Could you check a few things on this model? Use its own coordinates, in mm. Face numbers are marked on the shaded views. A direction names the side the tool comes from. Round coordinates to 2 decimals unless told otherwise and drop trailing zeros. Write each loop counter-clockwise with the first axis right and the second up, starting at its lowest first coordinate (ties: lowest second). Pieces come first, ordered by that corner, then holes. Notation, with made-up numbers: (-30, 53) -> (-1, 53) arc R30 ccw to (-1, 83) -> close; hole circle Ø8 at (82.25, -32.75). An arc over 180 degrees is marked (long way). Answer in a Markdown table with one row per item.
from build123d import *

# Parameters (mm, degrees)
BOSS_EXTRU_1_DEPTH      = 2
ESQUISSE3_R             = 1.5
ENL_V_MAT_EXTRU_1_DEPTH = 2
BOSS_EXTRU_2_START      = -2
ESQUISSE4_R             = 1.4
BOSS_EXTRU_2_DEPTH      = 2
ESQUISSE5_R             = 1.6
BOSS_EXTRU_3_DEPTH      = 1
ESQUISSE6_W             = 4
ESQUISSE6_H             = 1
ENL_V_MAT_EXTRU_2_DEPTH = 3


with BuildPart() as part:
    # Esquisse2 → Boss.-Extru.1 (new body)
    with BuildSketch(Plane.XY):
        with BuildLine():
            Line((-2.010396268, -6.486037297), (-15.087524479, 11.205449858))
            ThreePointArc((-15.087524479, 11.205449858), (-14.563165508, 14.701883422), (-11.066731944, 14.177524451))
            Line((-11.066731944, 14.177524451), (2.010396268, -3.513962703))
            ThreePointArc((2.010396268, -3.513962703), (1.486037297, -7.010396268), (-2.010396268, -6.486037297))
        make_face()
    extrude(amount=BOSS_EXTRU_1_DEPTH)

    # Esquisse3 → Enlèv. mat.-Extru.1 (cut)
    with BuildSketch(Plane.XY.offset(2)):
        with Locations((0, -5)):
            Circle(ESQUISSE3_R)
    extrude(amount=-ENL_V_MAT_EXTRU_1_DEPTH, mode=Mode.SUBTRACT)

    # Esquisse4 → Boss.-Extru.2 (add)
    with BuildSketch(Plane.XY.offset(2).offset(BOSS_EXTRU_2_START)):
        with Locations((-13.077128211, 12.691487155)):
            Circle(ESQUISSE4_R)
    extrude(amount=-BOSS_EXTRU_2_DEPTH)

    # Esquisse5 → Boss.-Extru.3 (add)
    with BuildSketch(Plane(origin=(0, 0, -2), x_dir=(-1, 0, 0), z_dir=(0, 0, -1))):
        with Locations((13.077128211, 12.691487155)):
            Circle(ESQUISSE5_R)
    extrude(amount=BOSS_EXTRU_3_DEPTH)

    # Esquisse6 → Enlèv. mat.-Extru.2 (cut)
    with BuildSketch(Plane(origin=(0, 0, -3), x_dir=(-1, 0, 0), z_dir=(0, 0, -1))):
        with Locations((13.077128211, 12.691487155)):
            Rectangle(ESQUISSE6_W, ESQUISSE6_H)
    extrude(amount=-ENL_V_MAT_EXTRU_2_DEPTH, mode=Mode.SUBTRACT)


solid = part.part
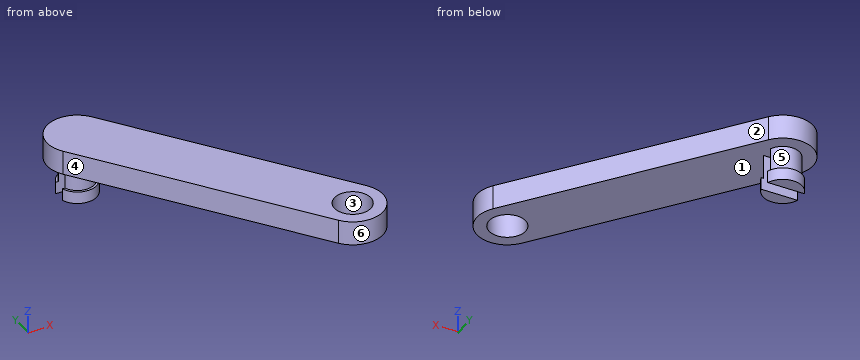
1) Please list where these lines run through material, in increasing order: line 1 (Z direction, x = -5.5, y = 0); line 2 (Y direction, x = 0, z = 1.15); line 3 (Y direction, x = -12, z = -0.95).
Findings:
| item | result |
|---|---|
| line 1 | z = 0 to 2 |
| line 2 | y = -7.5 to -6.5, -3.5 to -0.79 |
| line 3 | y = 11.8 to 12.19, 13.19 to 13.59 |
2) Imagine slicing it at D-D, the plane y = 11.75. Please give me the cut outline in (x, z).
Findings:
| item | result |
|---|---|
| outline | (-15.39, 0) -> (-14.11, 0) -> (-14.11, -2) -> (-14.37, -2) -> (-14.37, -3) -> (-11.78, -3) -> (-11.78, -2) -> (-12.04, -2) -> (-12.04, 0) -> (-9.27, 0) -> (-9.27, 2) -> (-15.39, 2) -> close |
3) For the marked faces 5 and 6, which set-ups out of +Z, -Z, +X, -X, +Y, -Y let a thin tool reach every point of the face, with its end or its side?
Findings:
| item | result |
|---|---|
| face 5 | +Y |
| face 6 | +Z, -Z |
4) Thinking about a two-plate mould opening in X: for the marked faces 1, 2, 3 and 4, which applies, +X half, -X half, draft (parallel to the pull), parting line (faces both ways), or undercut?
Findings:
| item | result |
|---|---|
| face 1 | draft |
| face 2 | +X half |
| face 3 | undercut |
| face 4 | -X half |
5) Imagine slicing it at B-B, the plane x = 0. Please give me the cut outline in (y, z).
Findings:
| item | result |
|---|---|
| outline | (-7.5, 0) -> (-6.5, 0) -> (-6.5, 2) -> (-7.5, 2) -> close; (-3.5, 0) -> (-0.79, 0) -> (-0.79, 2) -> (-3.5, 2) -> close |
6) Imagine slicing it at C-C, the plane z = -1.5. Please give me the cut outline in (x, y), plus the area to 3 significant figures.
Findings:
| item | result |
|---|---|
| outline | (-14.38, 12.19) arc R1.4 ccw to (-11.77, 12.19) -> close; (-14.38, 13.19) -> (-11.77, 13.19) arc R1.4 ccw to start |
| area | 3.42 mm^2 |
7) Imagine slicing it at A-A, the plane y = -5. Please give me the cut outline in (x, z).
Findings:
| item | result |
|---|---|
| outline | (-3.11, 0) -> (-1.5, 0) -> (-1.5, 2) -> (-3.11, 2) -> close; (1.5, 0) -> (2.5, 0) -> (2.5, 2) -> (1.5, 2) -> close |
8) For pin 1 (1 mm diameter, centred on x = -5.5, y = 10, fed in from +Z); pin 2 (5.5 mm diameter, centred on x = -9.5, y = 4.5, fed in from -Z); pin 3 (1 mm diameter, centred on y = -0.5, z = 0.5, fed in from +X); pin 4 (1.5 mm diameter, centred on x = -13, z = -2, fed in from -Y), each with a flat end and sliding along its axis, tell me the tip position at first contact or that it passes through.
Findings:
| item | result |
|---|---|
| pin 1 | passes through |
| pin 2 | stops at z = 0 |
| pin 3 | stops at x = 0.15 |
| pin 4 | stops at y = 11.09 |
